Autodesk Fusion 360 part; units mm, degrees
sketch "Sketch1" plane through (0, 0, 0) normal (0, 0, 1) x (1, 0, 0)
  line L0 (-30.5, 32.5) -> (30.5, 32.5)
  line L1 (32.5, 30.5) -> (32.5, -30.5)
  line L2 (30.5, -32.5) -> (-30.5, -32.5)
  line L3 (-32.5, -30.5) -> (-32.5, 30.5)
  line L4 (-32.5, 32.5) -> (32.5, -32.5) construction
  line L5 (32.5, 32.5) -> (-32.5, -32.5) construction
  circle A0 centre (0, 0) radius 2.5
  circle A1 centre (0, 10) radius 2.5
  circle A2 centre (0, 20) radius 3.5
  circle A3 centre (0, -10) radius 2.5
  circle A4 centre (0, -20) radius 2.5
  circle A5 centre (10, -20) radius 2.5
  circle A6 centre (10, 0) radius 2.5
  circle A7 centre (10, 20) radius 2.5
  circle A8 centre (20, -20) radius 2.5
  circle A9 centre (20, 20) radius 2.5
  line L6 (17.5, 10) -> (17.5, -10)
  line L7 (22.5, -10) -> (22.5, 10)
  arc A10 (22.5, 10) -> (17.5, 10) centre (20, 10) ccw
  arc A11 (17.5, -10) -> (22.5, -10) centre (20, -10) ccw
  line L8 (29, 3) -> (29, -3)
  line L9 (26, -3) -> (26, 3)
  arc A12 (29, 3) -> (26, 3) centre (27.5, 3) ccw
  arc A13 (26, -3) -> (29, -3) centre (27.5, -3) ccw
  arc A14 (29, 23) -> (26, 23) centre (27.5, 23) ccw
  line L10 (29, 23) -> (29, 17)
  arc A15 (26, 17) -> (29, 17) centre (27.5, 17) ccw
  line L11 (26, 17) -> (26, 23)
  arc A16 (26, -23) -> (29, -23) centre (27.5, -23) ccw
  line L12 (29, -17) -> (29, -23)
  line L13 (26, -23) -> (26, -17)
  arc A17 (29, -17) -> (26, -17) centre (27.5, -17) ccw
  circle A18 centre (-10, -20) radius 2.5
  line L14 (-26, -3) -> (-26, 3)
  line L15 (-26, 17) -> (-26, 23)
  arc A19 (-29, -3) -> (-26, -3) centre (-27.5, -3) ccw
  circle A20 centre (-10, 20) radius 2.5
  circle A21 centre (-20, -20) radius 2.5
  line L16 (-29, 23) -> (-29, 17)
  circle A22 centre (-20, 20) radius 2.5
  arc A23 (-17.5, 10) -> (-22.5, 10) centre (-20, 10) ccw
  arc A24 (-26, 23) -> (-29, 23) centre (-27.5, 23) ccw
  arc A25 (-22.5, -10) -> (-17.5, -10) centre (-20, -10) ccw
  arc A26 (-26, 3) -> (-29, 3) centre (-27.5, 3) ccw
  line L17 (-17.5, 10) -> (-17.5, -10)
  line L18 (-29, 3) -> (-29, -3)
  circle A27 centre (-10, 0) radius 2.5
  arc A28 (-29, -23) -> (-26, -23) centre (-27.5, -23) ccw
  line L19 (-22.5, -10) -> (-22.5, 10)
  line L20 (-26, -23) -> (-26, -17)
  arc A29 (-26, -17) -> (-29, -17) centre (-27.5, -17) ccw
  arc A30 (-29, 17) -> (-26, 17) centre (-27.5, 17) ccw
  line L21 (-29, -17) -> (-29, -23)
  arc A31 (-30.5, 32.5) -> (-32.5, 30.5) centre (-30.5, 30.5) ccw
  arc A32 (32.5, 30.5) -> (30.5, 32.5) centre (30.5, 30.5) ccw
  arc A33 (30.5, -32.5) -> (32.5, -30.5) centre (30.5, -30.5) ccw
  arc A34 (-32.5, -30.5) -> (-30.5, -32.5) centre (-30.5, -30.5) ccw
  circle A35 centre (0, 20) radius 1.65
  circle A36 centre (0, 20) radius 3.35
  circle A37 centre (0, -20) radius 1.65
  circle A38 centre (0, -20) radius 2.35
  dimension "d1" = 65
  dimension "d2" = 65
  dimension "d3" = 5
  dimension "d8" = 7
  dimension "d11" = 0
  dimension "d12" = -10
  dimension "d13" = 5
  dimension "d14" = 5
  dimension "d16" = 5
  dimension "d17" = 3
  dimension "d19" = 3
  dimension "d20" = 3
  dimension "d21" = 3
  dimension "d22" = 3
  dimension "d23" = 3
  dimension "d24" = 2
  dimension "d25" = 2
  dimension "d26" = 2
  dimension "d27" = 2
  dimension "d42" = 3.3
  dimension "d43" = 6.7
  dimension "d44" = 3.3
  dimension "d45" = 4.7
ref_plane "WorkPlane1" through (0, 0, 3) normal (0, 0, 1) x (1, 0, 0)
sketch "Sketch3" plane through (0, 0, 3) normal (0, 0, 1) x (1, 0, 0)
  line L0 (13.5, 32.5) -> (-13.5, 32.5)
  line L1 (-13.5, 32.5) -> (-13.5, -32.5)
  line L2 (-13.5, -32.5) -> (13.5, -32.5)
  line L3 (13.5, -32.5) -> (13.5, 32.5)
  line L4 (13.5, 32.5) -> (-13.5, -32.5) construction
  line L5 (-13.5, 32.5) -> (13.5, -32.5) construction
  circle A0 centre (0, 20) radius 3.35
  circle A1 centre (0, -20) radius 2.35
  circle A2 centre (0, 20) radius 2.15
  circle A3 centre (0, -20) radius 1.65
  dimension "d33" = 27
  dimension "d34" = 65
  dimension "d67" = 6.7
  dimension "d68" = 4.7
  dimension "d69" = 4.3
  dimension "d70" = 3.3
ref_plane "WorkPlane2" through (0, 0, 12) normal (0, 0, 1) x (1, 0, 0)
sketch "Sketch4" plane through (0, 0, 12) normal (0, 0, 1) x (1, 0, 0)
  line L0 (16.5, 32.5) -> (-16.5, 32.5)
  line L1 (-16.5, 32.5) -> (-16.5, -32.5)
  line L2 (16.5, -32.5) -> (16.5, 32.5)
  line L3 (-16.5, -32.5) -> (-16.5, -62.5)
  line L4 (-16.5, -62.5) -> (16.5, -62.5)
  line L5 (16.5, -62.5) -> (16.5, -32.5)
  circle A0 centre (0, 20) radius 2.15
  circle A1 centre (0, -20) radius 1.65
  dimension "d38" = 30
  dimension "d39" = 33
ref_plane "WorkPlane3" through (0, 0, 14.8) normal (0, 0, 1) x (1, 0, 0)
sketch "Sketch5" plane through (0, 0, 14.8) normal (0, 0, 1) x (1, 0, 0)
  circle A0 centre (0, 20) radius 4.5
  circle A1 centre (0, -20) radius 4.5
  dimension "d61" = 9
  dimension "d62" = 9
extrude "Extrude8" add sketch "Sketch3" along normal blind 9 contours L0 L1 L2 L3 | A0 | A1 makes body 1
extrude "Extrude9" add sketch "Sketch4" along normal blind 2.8 bodies 1
extrude "Extrude10" cut sketch "Sketch5" against normal blind 4 bodies 1
extrude "Extrude11" add sketch "Sketch3" against normal blind 2 contours A0 bodies 1
fillet "Fillet3" radius 1 1 edges at (-3.1233, 21.2114, 1) on bodies 1
extrude "Extrude12" add sketch "Sketch3" against normal blind 1.5 contours A1 bodies 1
fillet "Fillet4" radius 0.5 1 edges at (-2.191, -19.1502, 1.5) on bodies 1
extrude "Extrude1" add sketch "Sketch1" along normal blind 3 separate body contours L0 L1 L2 L3 A31 A32 A33 A34 makes body 2
hidden bodies 2
equation "d43 = 7 mm - 0.3 mm"
equation "d45 = 5 mm - 0.3 mm"
equation "d67 = 7 mm - 0.3 mm"
equation "d68 = 5 mm - 0.3 mm"
Read the model definition and answer for the solid it produces. Units are mm, in the model's axes. A direction names the side the tool comes from. Round coordinates to 2 decimals unless told otherwise and drop trailing zeros. Write each loop counter-clockwise with the first axis right and the second up, starting at its lowest first coordinate (ties: lowest second). Pieces come first, ordered by that corner, then holes. Notation, with made-up numbers: (81.25, 8.25) - (135.25, 8.25) arc R19 cw to (135.25, 21.25) - close; hole circle Ø4 at (52.25, 5.25). An arc over 180 degrees is marked (long way). Use a Markdown table: item, result.
(1) Each of these flat-tipped pins is pushed along its axis until it touches: pin 1 Ø3 at (y, z) = (-23, 6.5) entering from +X; pin 2 Ø16.5 at (x, y) = (-3.5, 3.5) entering from -Z; pin 3 Ø4 at (x, y) = (0, -20.5) entering from -Z; pin 4 Ø14.5 at (x, y) = (0, 20) entering from +Z. Where does it stop, or does it pass through?
Reported:
| item | result |
|---|---|
| pin 1 | x = 13.5 |
| pin 2 | z = 3 |
| pin 3 | z = 1.5 |
| pin 4 | z = 14.8 |
(2) Straight lines are drawn through the part: line 1 along Y through (x, z) = (0, 8); line 2 along Y through (x, z) = (0, 12.8); line 3 along X through (y, z) = (-20, 8). For each, find the intervals that lie inside material, in ascending order. Write a range as [from, to].
Reported:
| item | result |
|---|---|
| line 1 | [-32.5, -21.65], [-18.35, 17.85], [22.15, 32.5] |
| line 2 | [-62.5, -24.5], [-15.5, 15.5], [24.5, 32.5] |
| line 3 | [-13.5, -1.65], [1.65, 13.5] |
(3) The part is cut by section D-D (y = -20). Write down the section's boundary in (x, z).
Reported:
| item | result |
|---|---|
| outline | (-16.5, 12) - (-13.5, 12) - (-13.5, 3) - (-2.35, 3) - (-2.35, 2) arc R0.5 ccw to (-1.85, 1.5) - (-1.65, 1.5) - (-1.65, 10.8) - (-4.5, 10.8) - (-4.5, 14.8) - (-16.5, 14.8) - close; (1.65, 1.5) - (1.85, 1.5) arc R0.5 ccw to (2.35, 2) - (2.35, 3) - (13.5, 3) - (13.5, 12) - (16.5, 12) - (16.5, 14.8) - (4.5, 14.8) - (4.5, 10.8) - (1.65, 10.8) - close |
(4) Which of the six approach directions +Z, -Z, +X, -X, +Y, -Y give full straight-line access (tool end or side, diameter ignored) to faces 1 (the flat face through (13.5, 0, 7)), 2 (the cylindrical face through (2.419, 23.794, 12.828)), 3 (the flat face through (0, -32.5, 7)), 4 (the cylindrical face through (-0.44, 23.32, 2.51))?
Reported:
| item | result |
|---|---|
| face 1 | -Z, +X, +Y, -Y |
| face 2 | +Z |
| face 3 | -Z, +X, -X, -Y |
| face 4 | -Z |
(5) The mould has two halves that part along Y. Classify faces 5 (the cylindrical face through (-0.215, -21.636, 6.085)), 6 (the flat face through (-13.5, 0, 7)), 7 (the flat face through (0, -62.5, 13)), 8 (the flat face through (0, -22, 10.8)): released by +Y, released by -Y, zero draft, split by the parting line, or undercut.
Reported:
| item | result |
|---|---|
| face 5 | undercut |
| face 6 | zero draft |
| face 7 | released by -Y |
| face 8 | undercut |
(6) The part is cut by section C-C (z = 13.5). Write down the section's boundary in (x, y).
Reported:
| item | result |
|---|---|
| outline | (-16.5, -62.5) - (16.5, -62.5) - (16.5, 32.5) - (-16.5, 32.5) - close; hole circle Ø9 at (0, -20); hole circle Ø9 at (0, 20) |
(7) The part is cut by section A-A (y = 20). Write down the section's boundary in (x, z), then the cut area to 3 significant figures.
Reported:
| item | result |
|---|---|
| outline | (-16.5, 12) - (-13.5, 12) - (-13.5, 3) - (-3.35, 3) - (-3.35, 2) arc R1 ccw to (-2.35, 1) - (-2.15, 1) - (-2.15, 10.8) - (-4.5, 10.8) - (-4.5, 14.8) - (-16.5, 14.8) - close; (2.15, 1) - (2.35, 1) arc R1 ccw to (3.35, 2) - (3.35, 3) - (13.5, 3) - (13.5, 12) - (16.5, 12) - (16.5, 14.8) - (4.5, 14.8) - (4.5, 10.8) - (2.15, 10.8) - close |
| area | 270 mm2 |
(8) The part is cut by section B-B (x = 0). State how many separate pieces and enclosed holes the cut face has, then the cut area to 3 significant figures.
Reported:
| item | result |
|---|---|
| separate pieces | 3 |
| enclosed holes | 0 |
| area | 726 mm2 |
